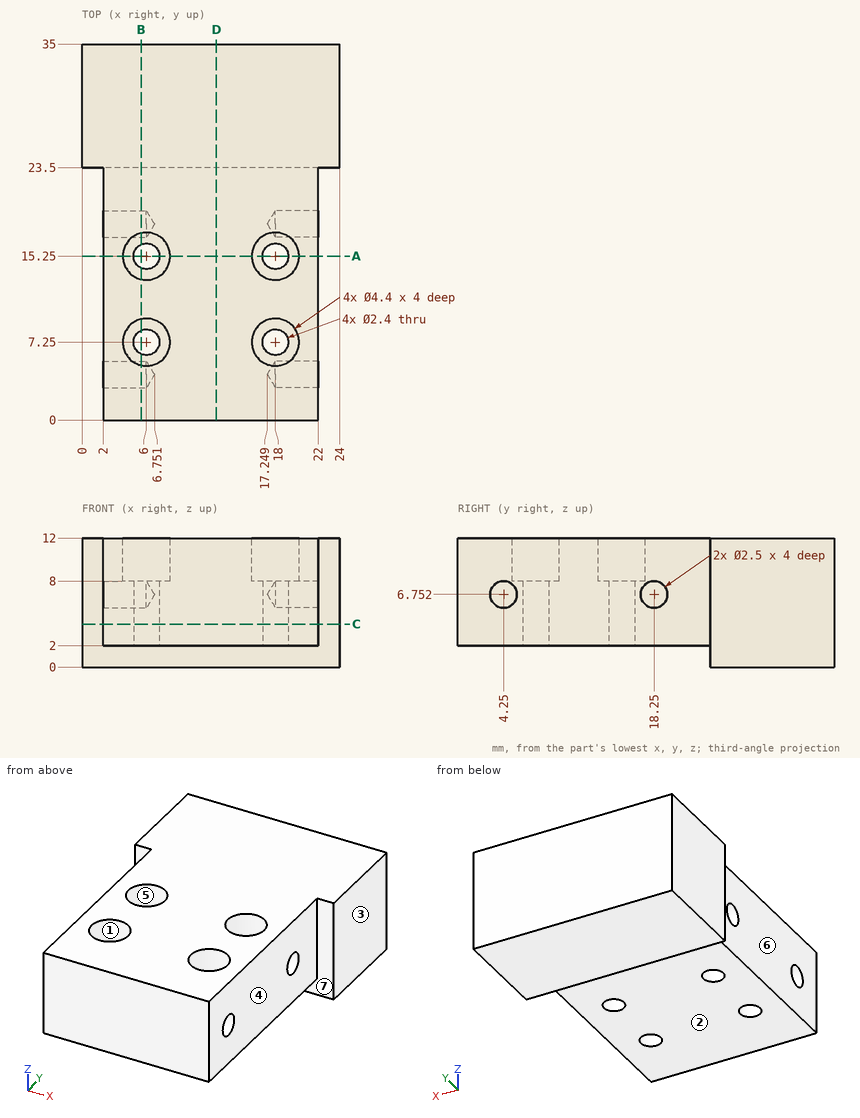
Verification items for this drawing (mm, ordinates from the low corner). A direction names the side the tool comes from. Give positions to 0.01 mm unless a question says otherwise; leave off trailing zeros. Loops run counter-clockwise (first coordinate to the right, second up) from the corner with the lowest first, then second, coordinate; pieces in that order, holes last. Notation, with made-up numbers: M 47.5,87 L 71.5,87 A22 ccw 71.5,112 Z; hole C -11.5,24 d8. An arc over 180 degrees is marked long. Answer as CSV lines item,"result".
Item 1: Access from +Z, -Z, +X, -X, +Y, -Y to the whole of each face (thin tool, end or side, straight path). Record for the marked faces 4, 5, 6 and 7.
Values:
face 4,"+Z, -Z, +X, -Y"
face 5,"+Z"
face 6,"+Z, -Z, -X, -Y"
face 7,"-Z, -Y"
Item 2: Depth check by flat-ended pin: P1, Ø3.5, axis at x = 18, y = 7.25, coming from the -Z side; P2, Ø2, axis at x = 7, y = 7, coming from the +Z side; P3, Ø1.5, axis at y = 18.25, z = 6.75, coming from the -X side. Enter the tip coordinate at first touch or a pass-through.
Values:
P1,"stops at z = 2"
P2,"stops at z = 8"
P3,"stops at x = 6.3"
Item 3: Cross-section at A-A on y = 15.25. Record the cut outline in (x, z).
Values:
outline,"M 2,2 L 4.8,2 L 4.8,8 L 3.8,8 L 3.8,12 L 2,12 Z; M 7.2,2 L 16.8,2 L 16.8,8 L 15.8,8 L 15.8,12 L 8.2,12 L 8.2,8 L 7.2,8 Z; M 19.2,2 L 22,2 L 22,12 L 20.2,12 L 20.2,8 L 19.2,8 Z"
Item 4: Release check for a two-part mould opening along X. For the marked faces 1, 2 and 3 record: pulls with the +X half, pulls with the -X half, needs draft (parallel to the pull), parting line crosses it, or undercut.
Values:
face 1,"undercut"
face 2,"needs draft"
face 3,"pulls with the +X half"
Item 5: Cross-section at B-B on x = 5.5. Record the cut outline in (y, z).
Values:
outline,"M 0,2 L 6.16,2 L 6.16,8 L 5.11,8 L 5.11,12 L 0,12 Z; M 8.34,2 L 14.16,2 L 14.16,8 L 13.11,8 L 13.11,12 L 9.39,12 L 9.39,8 L 8.34,8 Z; M 16.34,2 L 23.5,2 L 23.5,0 L 35,0 L 35,12 L 17.39,12 L 17.39,8 L 16.34,8 Z; hole C 4.25,6.75 d2.5; hole C 18.25,6.75 d2.5"
Item 6: Cross-section at D-D on x = 12.5. Record the cut outline in (y, z), and give its area (3 significant figures).
Values:
outline,"M 0,2 L 23.5,2 L 23.5,0 L 35,0 L 35,12 L 0,12 Z"
area,"373 mm²"
Item 7: Material ranges on line 1 (Y direction, x = 6, z = 9); line 2 (Y direction, x = 6, z = 4.1); line 3 (X direction, y = 5.5, z = 9.75), recorded low to high.
Values:
line 1,"y = 0 to 5.05, 9.45 to 13.05, 17.45 to 35"
line 2,"y = 0 to 6.05, 8.45 to 14.05, 16.45 to 35"
line 3,"x = 2 to 4.67, 7.33 to 16.67, 19.33 to 22"
Item 8: Cross-section at C-C on z = 4. Record the cut outline in (x, y).
Values:
outline,"M 0,23.5 L 2,23.5 L 2,0 L 22,0 L 22,23.5 L 24,23.5 L 24,35 L 0,35 Z; hole C 6,7.25 d2.4; hole C 6,15.25 d2.4; hole C 18,7.25 d2.4; hole C 18,15.25 d2.4"
